Check sheet for the drawn part. Datum: minimum x, y, z corner. Units: mm. A direction names the side the tool comes from. Give positions to 0.01 mm unless a question says otherwise; leave off trailing zeros. Write each loop counter-clockwise with the first axis right and the second up, starting at its lowest first coordinate (ties: lowest second). Pieces come first, ordered by that corner, then holes. Notation, with made-up numbers: (44.25, -23) -> (61.25, -23) arc R25 cw to (61.25, 4) -> close; hole circle Ø6 at (24.5, 84.5). An arc over 180 degrees is marked (long way). Use CSV: the item, a comma, the result in double quotes. Start each with the question number.
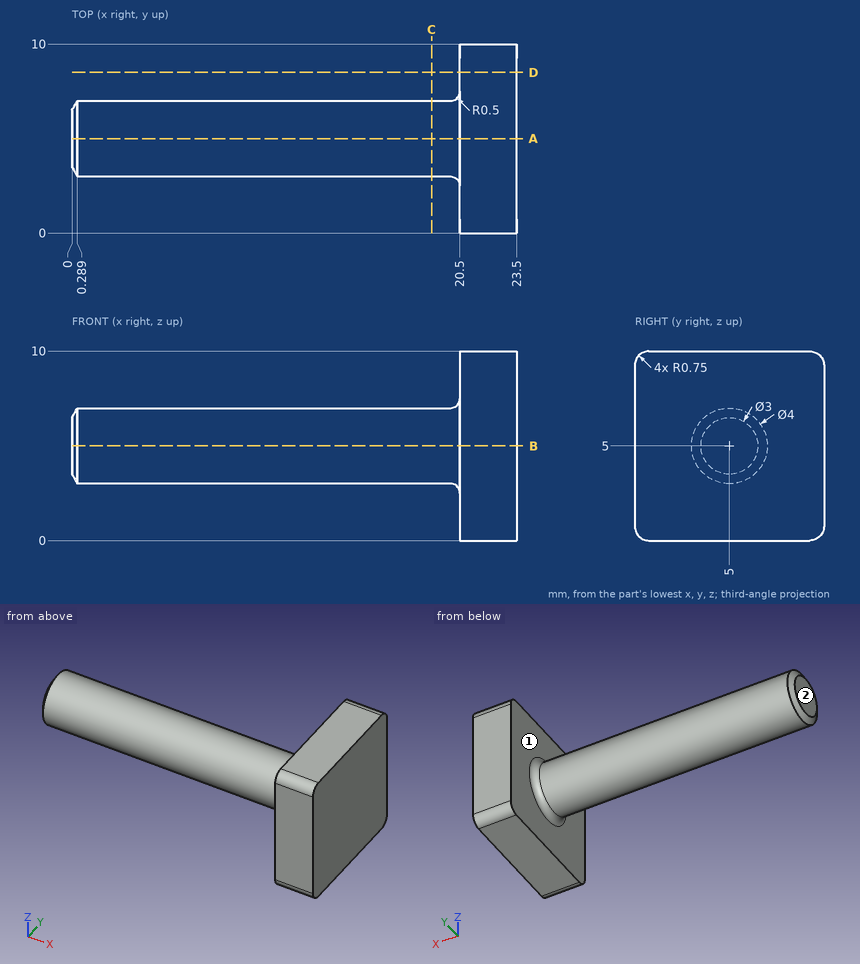
(1) Section check A-A on y = 5. Record the cut outline in (x, z), then the cut area to 3 significant figures.
(2) Set-up check for the marked faces 1 and 2: record each of +Z, -Z, +X, -X, +Y, -Y from which the full face is reachable in a straight line by a thin tool's end or side.
(3) Section check C-C on x = 19. Record the cut outline in (y, z), then the cut area to 3 significant figures.
(4) Section check D-D on y = 8.5. Record the cut outline in (x, z).
(5) Thickness scan on line 1 (X direction, y = 8.5, z = 5.25); line 2 (Z direction, x = 10.5, y = 5); line 3 (Z direction, x = 16, y = 3.75). Record the ranges inside material, lowest first. Write a range as from..to.
(6) Go/stop test with flat-tipped pins: pin 1 (4 mm diameter, centred on x = 3, y = 2, fed in from -Z); pin 2 (1 mm diameter, centred on x = 15, y = 1, fed in from +Z); pin 3 (4 mm diameter, centred on x = 11, y = 7, fed in from -Z). Record where each tip stops, or that it passes through.
Data:
1,outline,"(0, 3.5) -> (0.29, 3) -> (20, 3) arc R0.5 cw to (20.5, 2.5) -> (20.5, 0) -> (23.5, 0) -> (23.5, 10) -> (20.5, 10) -> (20.5, 7.5) arc R0.5 cw to (20, 7) -> (0.29, 7) -> (0, 6.5) -> close"
1,area,"112 mm2"
2,face 1,"-X"
2,face 2,"+Z, -Z, -X, +Y, -Y"
3,outline,"circle Ø4 at (5, 5)"
3,area,"12.6 mm2"
4,outline,"(20.5, 0) -> (23.5, 0) -> (23.5, 10) -> (20.5, 10) -> close"
5,line 1,"x = 20.5..23.5"
5,line 2,"z = 3..7"
5,line 3,"z = 3.44..6.56"
6,pin 1,"stops at z = 3.27"
6,pin 2,"passes through"
6,pin 3,"stops at z = 3"
